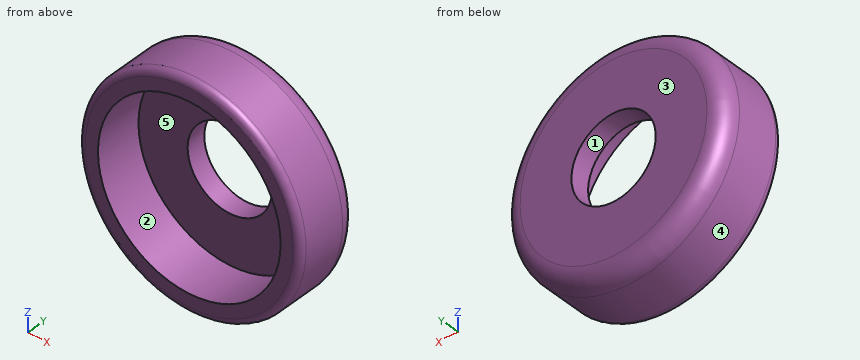
from build123d import *

# Parameters (mm, degrees)
FILLET1_R          = 1.5875
SKETCH2_R          = 3.81
CUT_EXTRUDE1_DEPTH = 16.442907563
FILLET2_R          = 0.635


with BuildPart() as part:
    # Sketch1 → Base-Revolve (revolve)
    with BuildSketch(Plane.XY, mode=Mode.PRIVATE) as base_revolve_sk:
        Polygon((-8.255, 0), (-10.033, 0), (-10.033, 6.096), (0, 6.096), (0, 4.318), (-8.255, 4.318), align=None)
    revolve(base_revolve_sk.sketch.rotate(Axis((0, 0, 0), (0, 1, 0)), 270), axis=Axis((0, 0, 0), (0, 1, 0)))

    # Fillet1
    fillet1_edges = [part.edges().sort_by_distance(p)[0] for p in [
        (0, 6.096, 10.033),
    ]]
    fillet(fillet1_edges, radius=FILLET1_R)

    # Sketch2 → Cut-Extrude1 (cut, through all)
    with BuildSketch(Plane(origin=(0, 6.096, 0), x_dir=(-1, 0, 0), z_dir=(0, 1, 0))):
        with Locations(Location((0, 0, 0), (0, 0, 90))):
            Circle(SKETCH2_R)
    extrude(amount=-CUT_EXTRUDE1_DEPTH, mode=Mode.SUBTRACT)

    # Fillet2
    fillet2_edges = [part.edges().sort_by_distance(p)[0] for p in [
        (0, 0, 10.033),
    ]]
    fillet(fillet2_edges, radius=FILLET2_R)


solid = part.part
Can you work these out from the model? Positions are in its coordinate system, mm. Face numbers are marked on the shaded views. A direction names the side the tool comes from. Give positions to 0.01 mm unless a question says otherwise; leave off trailing zeros. Order: outer loops, then holes, each group sorted by start corner. A loop starts at its lowest first (then second) coordinate and runs counter-clockwise, first axis right, second up. Notation, with made-up numbers: (16.5, 20.25) - (27.5, 20.25) arc R21 cw to (27.5, 40.25) - close; hole circle Ø7 at (54, 42). An arc over 180 degrees is marked (long way). Write each question's results on one line, items separated by ' | '.
1) Suppose I cut it at A-A, the plane z = 0. Write out the boundary of the cut face in (x, y) (1 decimal).
Final values:
outline: (-10, 0.6) arc R0.6 ccw to (-9.4, 0) - (-8.3, 0) - (-8.3, 4.3) - (-3.8, 4.3) - (-3.8, 6.1) - (-8.4, 6.1) arc R1.6 ccw to (-10, 4.5) - close; (3.8, 4.3) - (8.3, 4.3) - (8.3, 0) - (9.4, 0) arc R0.6 ccw to (10, 0.6) - (10, 4.5) arc R1.6 ccw to (8.4, 6.1) - (3.8, 6.1) - close
2) Suppose I cut it at B-B, the plane x = 0. Write out the boundary of the cut face in (y, z) (1 decimal).
Final values:
outline: (0, -9.4) arc R0.6 ccw to (0.6, -10) - (4.5, -10) arc R1.6 ccw to (6.1, -8.4) - (6.1, -3.8) - (4.3, -3.8) - (4.3, -8.3) - (0, -8.3) - close; (0, 8.3) - (4.3, 8.3) - (4.3, 3.8) - (6.1, 3.8) - (6.1, 8.4) arc R1.6 ccw to (4.5, 10) - (0.6, 10) arc R0.6 ccw to (0, 9.4) - close
3) On a 3-axis mill with a long thin cutter (end or side, diameter ignored), from which of +Z, -Z, +X, -X, +Y, -Y can I reach the whole of each face in a straight line? I mean the marked faces 1 and 2. Say none if no direction works.
Final values:
face 1: +Y, -Y | face 2: -Y
4) I'm going to push flat-ended pins straight in: pin 1 Ø9 at (x, z) = (0, 0) entering from -Y; pin 2 Ø3 at (x, y) = (5.5, 1.5) entering from -Z; pin 3 Ø1 at (x, y) = (-3.5, 5) entering from +Z. Where does each tip first touch, or does it pass through?
Final values:
pin 1: stops at y = 4.32 | pin 2: stops at z = -9.2 | pin 3: stops at z = 9.53
5) If we mould it in two halves opening along Z, with no side actions, what happens to the marked faces 3, 4 and 5? For each: pulls with the +Z half, pulls with the -Z half, needs draft (parallel to the pull), parting line crosses it, or undercut.
Final values:
face 3: needs draft | face 4: parting line crosses it | face 5: undercut
6) Please list where these lines run through material, in increasing order: line 1 along X through (y, z) = (2.1, 0) (3 decimals); line 2 along X through (y, z) = (3, 3.75); line 3 along Y through (x, z) = (6.25, -1.25). Write a range as [from, to].
Final values:
line 1: x = [-10.033, -8.255], [8.255, 10.033] | line 2: x = [-9.31, -7.35], [7.35, 9.31] | line 3: y = [4.32, 6.1]
7) Suppose I cut it at C-C, the plane y = 2. Write out the boundary of the cut face in (x, z) (3 decimals), then the cut area to 3 significant figures.
Final values:
outline: circle Ø20.066 at (0, 0); hole circle Ø16.51 at (0, 0) | area: 102 mm^2
